For this review, use the dimensioned drawing (mm, ordinates from the lowest corner) and the shaded views. Give positions to 0.01 mm unless a question says otherwise; leave off trailing zeros. Loops run counter-clockwise (first coordinate to the right, second up) from the corner with the lowest first, then second, coordinate; pieces in that order, holes last. Notation, with made-up numbers: M -17.5,31 L 4.5,31 A17 ccw 4.5,40 Z; hole C -22.5,88 d1. An arc over 180 degrees is marked long. Use CSV: the item, a comma, the result in double quotes.
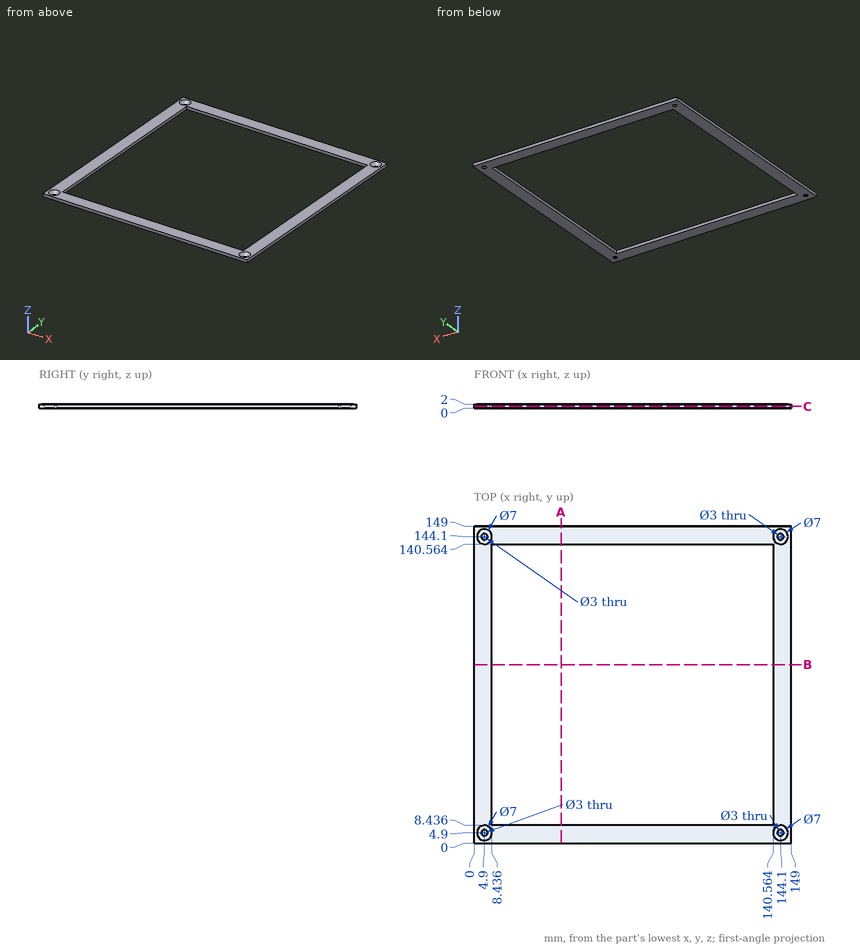
(1) Wall thickness on line 1 along Y through (x, z) = (12.5, 1) (1 decimal); line 2 along Y through (x, z) = (144.1, 0.05): over which ranges is each line inside the solid? List them lowest first. Write a range as [from, to].
A:
line 1,"[0, 8.4], [140.6, 149]"
line 2,"[0, 3.35], [6.45, 142.55], [145.65, 149]"
(2) We need section C-C on z = 0.9. State the section outline as (x, y) points (1 decimal).
A:
outline,"M 0,0 L 149,0 L 149,149 L 0,149 Z; hole C 4.9,4.9 d4.8; hole C 4.9,144.1 d4.8; hole M 8.4,8.4 L 140.6,8.4 L 140.6,140.6 L 8.4,140.6 Z; hole C 144.1,4.9 d4.8; hole C 144.1,144.1 d4.8"
(3) We need section A-A on x = 41. State the section outline as (y, z) points (1 decimal).
A:
outline,"M 0,0 L 8.4,0 L 8.4,2 L 0,2 Z; M 140.6,0 L 149,0 L 149,2 L 140.6,2 Z"
